```python
from build123d import *

# Parameters (mm, degrees)
CROQUIS1_W                 = 222
CROQUIS1_H                 = 30
CROQUIS1_R                 = 5
SALIENTE_EXTRUIR1_DEPTH    = 70
CORTAR_EXTRUIR1_DEPTH      = 30
CORTAR_EXTRUIR1_DEPTH_BACK = 30
CROQUIS2_R                 = 40
CROQUIS3_W                 = 142
CROQUIS3_H                 = 60
CORTAR_EXTRUIR2_DEPTH      = 201.889443058


with BuildPart() as part:
    # Croquis1 → Saliente-Extruir1 (new body)
    with BuildSketch(Plane(origin=(0, 0, 0), x_dir=(1, 0, 0), z_dir=(0, 1, 0))):
        with Locations((74.893970672, 3.671875)):
            Rectangle(CROQUIS1_W, CROQUIS1_H)
        with Locations(Location((-26.106029328, 3.671875, 0), (0, 0, 270))):
            Circle(CROQUIS1_R, mode=Mode.SUBTRACT)
        with Locations(Location((175.893970672, 3.671875, 0), (0, 0, 270))):
            Circle(CROQUIS1_R, mode=Mode.SUBTRACT)
    extrude(amount=SALIENTE_EXTRUIR1_DEPTH)

    # Croquis2 → Cortar-Extruir1 (cut, two sides: drawn at the far end of the back side and taken through both)
    with BuildSketch(Plane(origin=(0, 35, 0), x_dir=(-1, 0, 0), z_dir=(0, -1, 0)).offset(-CORTAR_EXTRUIR1_DEPTH_BACK)):
        with Locations((42.379372645, -2.333916419)):
            Circle(CROQUIS2_R)
        with Locations((-194.158036126, -5.581508709)):
            Circle(CROQUIS2_R)
    extrude(amount=CORTAR_EXTRUIR1_DEPTH + CORTAR_EXTRUIR1_DEPTH_BACK, mode=Mode.SUBTRACT)

    # Croquis3 → Cortar-Extruir2 (cut, through all)
    with BuildSketch(Plane.XY.offset(11.328125)):
        with Locations((74.893970672, 35)):
            Rectangle(CROQUIS3_W, CROQUIS3_H)
    extrude(amount=-CORTAR_EXTRUIR2_DEPTH, mode=Mode.SUBTRACT)


solid = part.part
```
Could you check a few things on this model? Use its own coordinates, in mm. A direction names the side the tool comes from. Coordinates: 2 decimals unless noted, no trailing zeros. Order: outer loops, then holes, each group sorted by start corner. A loop starts at its lowest first (then second) coordinate and runs counter-clockwise, first axis right, second up. Notation, with made-up numbers: M 53,14.25 L 81,14.25 A20 ccw 81,43.25 Z; hole C -16.75,65.25 d5. An arc over 180 degrees is marked long. Use a Markdown table: item, result. Add a question column.
Q1. If I drill on L1, parallel to Y at x = 70, z = 4; L2, parallel to X at y = 6.5, z = 2.5; L3, parallel to X at y = 13, z = 7, over which ranges is the centre line in solid material (lowest first)?
Q2. I want a section at A-A on z = -3.5. Give the number of separate pieces and of enclosed holes in the cut face, then the cut area to 3 significant figures.
Q3. I want a section at C-C on y = 41. List the corners of the cut face in (x, z) for me, then the cut area to 3 significant figures.
Q4. I want a section at D-D on z = -13.5. List the corners of the cut face in (x, y) for me.
Q5. I want a section at B-B on x = 69. List the corners of the cut face in (y, z) for me, then the cut area to 3 significant figures.
Q6. Which directions (+Z, -Z, +X, -X, +Y, -Y) give clear straight access to the entire face, cutting with the end or side of a thin tool? Please do faces 4 (the cylindrical face through (155.383, 35.42, -4.24)), 5 (the cylindrical face through (-30.987, 2.465, -4.756)), 6 (the flat face through (145.894, 35, -3)).
Q7. We'd pull the mould along Z, two halves only. Please class faces 1 (the flat face through (74, 5, -3)), 2 (the flat face through (73, 66, -18.672)), 3 (the cylindrical face through (-2.946, 35.42, -4.374)): pulls with the +Z half, pulls with the -Z half, needs draft (parallel to the pull), parting line crosses it, or undercut.
Q8. I'm going to push flat-ended pins straight in: pin 1 (8 mm diameter, centred on x = -26.11, z = -3.67, fed in from +Y); pin 2 (15 mm diameter, centred on y = 30, z = 1, fed in from +X); pin 3 (6 mm diameter, centred on x = 163.5, y = 48.5, fed in from +Z); pin 4 (15 mm diameter, centred on y = 27.5, z = -8.5, fed in from -X). Where does each tip first touch, or does it pass through?
Checked values:
| question | item | result |
|---|---|---|
| 1 | L1 | 0 to 5, 65 to 70 |
| 1 | L2 | -2.38 to 3.89, 145.89 to 154.28 |
| 1 | L3 | -2.65 to 3.89, 145.89 to 154.18 |
| 2 | separate pieces | 5 |
| 2 | enclosed holes | 1 |
| 2 | area | 2,980 mm² |
| 3 | outline | M -8.34,-18.67 L 3.89,-18.67 L 3.89,11.33 L -3.4,11.33 A40 cw Z; M 145.89,-18.67 L 162.35,-18.67 A40 cw 154.57,11.33 L 145.89,11.33 Z |
| 3 | area | 544 mm² |
| 4 | outline | M -36.11,0 L 185.89,0 L 185.89,5 L 159,5 L 159,65 L 185.89,65 L 185.89,70 L -36.11,70 L -36.11,65 L -5.65,65 L -5.65,5 L -36.11,5 Z; hole M 3.89,5 L 145.89,5 L 145.89,65 L 3.89,65 Z |
| 5 | outline | M 0,-18.67 L 5,-18.67 L 5,11.33 L 0,11.33 Z; M 65,-18.67 L 70,-18.67 L 70,11.33 L 65,11.33 Z |
| 5 | area | 300 mm² |
| 6 | face 4 | +X |
| 6 | face 5 | +Y, -Y |
| 6 | face 6 | +Z, -Z |
| 7 | face 1 | needs draft |
| 7 | face 2 | pulls with the -Z half |
| 7 | face 3 | undercut |
| 8 | pin 1 | through |
| 8 | pin 2 | x = 156.03 |
| 8 | pin 3 | z = -16.03 |
| 8 | pin 4 | x = -6.83 |
